Geometry: final body of the model. Coordinates: model frame, mm. Round coordinates to 2 decimals unless told otherwise and drop trailing zeros. Loops run counter-clockwise (first coordinate to the right, second up) from the corner with the lowest first, then second, coordinate; pieces in that order, holes last. Notation, with made-up numbers: (86.25, -3) -> (93.25, -3) arc R33 ccw to (93.25, 30) -> close; hole circle Ø1 at (52.25, -32). An arc over 180 degrees is marked (long way). Answer in a Markdown table with one row per item.
```python
from build123d import *

# Parameters (mm, degrees)
F1_DEPTH = 4.7


# Not quite as in the source:
# - ends of sketch curves that miss each other by under 0.0002 mm in the source are joined


with BuildPart() as f1:
    # F0 (on Right) → F1 (new body)
    with BuildSketch(Plane.YZ):
        with BuildLine():
            ThreePointArc((-1.2861936627, 9.5404589046), (-1.3764412196, 9.3943245755), (-1.4645028348, 9.2468626631))
            ThreePointArc((-1.4645028348, 9.2468626631), (-12.6873926867, 14.4502544968), (-22.1664207404, 6.501885459))
            ThreePointArc((-22.1664207404, 6.501885459), (-22.0324514747, -0.8678048449), (-17.463284327, -6.6516612154))
            add(Edge.make_bspline(
                [(-17.463284327, -6.6516612154), (-12.0709199928, -11.7001523748), (-6.6785564381, -16.7486430269), (-1.2861928833, -21.797133679)],
                knots=[0, 0, 0, 0, 22.160405753, 22.160405753, 22.160405753, 22.160405753], degree=3))
            add(Edge.make_bspline(
                [(14.8908962222, -6.6516617227), (9.4985326674, -11.7001523748), (4.1061691126, -16.7486430269), (-1.2861928833, -21.797133679)],
                knots=[0, 0, 0, 0, 22.160405753, 22.160405753, 22.160405753, 22.160405753], degree=3))
            ThreePointArc((14.8908962222, -6.6516617227), (19.4600641493, -0.8678048449), (19.594033415, 6.501885459))
            ThreePointArc((19.594033415, 6.501885459), (10.1150053613, 14.4502544968), (-1.1078844907, 9.2468626631))
            ThreePointArc((-1.1078844907, 9.2468626631), (-1.1959461058, 9.3943245755), (-1.2861936627, 9.5404589046))
        make_face()
    extrude(amount=F1_DEPTH)


solid = f1.part
```
Item 1: Cut plane B-B (z = -6). Output: boundary loops of the cut face in (x, y), then the cut area to 3 significant figures.
Answer:
| item | result |
|---|---|
| outline | (0, -18.37) -> (4.7, -18.37) -> (4.7, 15.79) -> (0, 15.79) -> close |
| area | 161 mm² |
Item 2: Line query: probe 1 along Y at (x, z) = (2.9, 10.5); probe 2 along Y at (x, z) = (2.55, 6.5); probe 3 along Y at (x, z) = (3.8, -16). Output: solid intervals per line, ascending. Write a range as [from, to].
Answer:
| item | result |
|---|---|
| probe 1 | y = [-19.95, -2.39], [-0.18, 17.38] |
| probe 2 | y = [-22.17, 19.59] |
| probe 3 | y = [-7.48, 4.91] |
Item 3: Pin query (flat end, axial travel): pin 1 Ø1.5 at (x, z) = (3, 5) entering from -Y. Return the tip coordinate at first contact, or that it passes through.
Answer:
| item | result |
|---|---|
| pin 1 | stops at y = -22.64 |
Item 4: Cut plane A-A (z = 10.5). Output: boundary loops of the cut face in (x, y), then the cut area to 3 significant figures.
Answer:
| item | result |
|---|---|
| outline | (0, -19.95) -> (4.7, -19.95) -> (4.7, -2.39) -> (0, -2.39) -> close; (0, -0.18) -> (4.7, -0.18) -> (4.7, 17.38) -> (0, 17.38) -> close |
| area | 165 mm² |
Item 5: Cut plane C-C (y = 16). Output: boundary loops of the cut face in (x, z).
Answer:
| item | result |
|---|---|
| outline | (0, -5.83) -> (4.7, -5.83) -> (4.7, 11.86) -> (0, 11.86) -> close |
